```python
from build123d import *

# Parameters (mm, degrees)
SKETCH1_W             = 90
SKETCH1_H             = 90
SKETCH1_R             = 34
BOSS_EXTRUDE1_DEPTH   = 24
SKETCH2_R             = 40.5
CUT_EXTRUDE1_DEPTH    = 16
SKETCH3_R             = 12.7
CUT_EXTRUDE2_DEPTH    = 19
M6X1_0_TAPPED_HOLE1_D = 5
FILLET1_R             = 5
SKETCH7_R             = 30
SKETCH7_R_2           = 20
SKETCH7_R_3           = 12.7
CUT_EXTRUDE3_DEPTH    = 66.620118866
SKETCH8_W             = 13.825432395
SKETCH8_H             = 1
SKETCH8_W_2           = 1
SKETCH8_H_2           = 13.825432395
CUT_EXTRUDE4_DEPTH    = 16


with BuildPart() as part:
    # Sketch1 → Boss-Extrude1 (new body)
    # profile 1 of 2: a face of its own
    with BuildSketch(Plane(origin=(0, 0, 0), x_dir=(1, 0, 0), z_dir=(0, 1, 0))):
        Rectangle(SKETCH1_W, SKETCH1_H)
        Circle(SKETCH1_R, mode=Mode.SUBTRACT)
    # profile 2 of 2: a face of its own
    with BuildSketch(Plane(origin=(0, 0, 0), x_dir=(1, 0, 0), z_dir=(0, 1, 0))):
        Circle(SKETCH1_R)
    extrude(amount=BOSS_EXTRUDE1_DEPTH)

    # Sketch2 → Cut-Extrude1 (cut)
    with BuildSketch(Plane(origin=(0, 24, 0), x_dir=(1, 0, 0), z_dir=(0, 1, 0))):
        with Locations(Location((0, 0, 0), (0, 0, 270))):
            Circle(SKETCH2_R)
    extrude(amount=-CUT_EXTRUDE1_DEPTH, mode=Mode.SUBTRACT)

    # Sketch3 → Cut-Extrude2 (cut)
    with BuildSketch(Plane(origin=(0, 8, 0), x_dir=(1, 0, 0), z_dir=(0, 1, 0))):
        with Locations(Location((0, 0, 0), (0, 0, 270))):
            Circle(SKETCH3_R)
    extrude(amount=-CUT_EXTRUDE2_DEPTH, mode=Mode.SUBTRACT)

    # M6x1.0 Tapped Hole1 (through all)
    with Locations(Plane(origin=(0, 0, 0), x_dir=(-1, 0, 0), z_dir=(0, -1, 0))):
        with Locations((35, 35), (35, -35), (-35, -35), (-35, 35)):
            Hole(M6X1_0_TAPPED_HOLE1_D / 2)

    # Fillet1
    fillet1_edges = [part.edges().sort_by_distance(p)[0] for p in [
        (-45, 12, 45),
        (-45, 12, -45),
        (45, 12, -45),
        (45, 12, 45),
    ]]
    fillet(fillet1_edges, radius=FILLET1_R)

    # Sketch7 → Cut-Extrude3 (cut, through all)
    # profile 1 of 2: a face of its own
    with BuildSketch(Plane(origin=(0, 8, 0), x_dir=(1, 0, 0), z_dir=(0, 1, 0))):
        with Locations(Location((0, 0, 0), (0, 0, 270))):
            Circle(SKETCH7_R)
        Circle(SKETCH7_R_2, mode=Mode.SUBTRACT)
    # profile 2 of 2: a face of its own
    with BuildSketch(Plane(origin=(0, 8, 0), x_dir=(1, 0, 0), z_dir=(0, 1, 0))):
        Circle(SKETCH7_R_2)
        Circle(SKETCH7_R_3, mode=Mode.SUBTRACT)
    extrude(amount=-CUT_EXTRUDE3_DEPTH, mode=Mode.SUBTRACT)

    # Sketch8 → Cut-Extrude4 (cut)
    with BuildSketch(Plane(origin=(0, 24, 0), x_dir=(1, 0, 0), z_dir=(0, 1, 0))):
        with Locations((42.446502967, 0)):
            Rectangle(SKETCH8_W, SKETCH8_H)
        with Locations((0, 42.446502967)):
            Rectangle(SKETCH8_W_2, SKETCH8_H_2)
        with Locations((0, -42.446502967)):
            Rectangle(SKETCH8_W_2, SKETCH8_H_2)
        with Locations((-42.446502967, 0)):
            Rectangle(SKETCH8_W, SKETCH8_H)
    extrude(amount=-CUT_EXTRUDE4_DEPTH, mode=Mode.SUBTRACT)


solid = part.part
```
The listing builds one solid part. Answer for the finished solid, in the listing's coordinates (mm). A direction names the side the tool comes from. Coordinates: 2 decimals unless noted, no trailing zeros. Loops run counter-clockwise (first coordinate to the right, second up) from the corner with the lowest first, then second, coordinate; pieces in that order, holes last. Notation, with made-up numbers: M -14,85.25 L 36,85.25 A26 ccw 36,117.25 Z; hole C 52,48 d2. An arc over 180 degrees is marked long. Answer as a JSON object with one key per item and string values. Group by question number.
Item 1: Each of these flat-tipped pins is pushed along its axis until it touches: P1, Ø1.4, axis at x = 44, y = 16, coming from the -Z side; P2, Ø3.5, axis at y = 13.5, z = -43.5, coming from the -X side; P3, Ø5, axis at x = -43.5, y = 19, coming from the +Z side. Where does it stop, or does it pass through?
Item 2: Section A-A (y = 21.75) is taken. Write down the section's boundary in (x, z).
Item 3: Section B-B (z = 27.5) is taken. Write down the section's boundary in (x, y).
Item 4: Determine the mould class of faces 1 (the face through (1.32, 4.06, -29.97)), 2 (the face through (43, 12, 44)), 3 (the face through (31, 24, -31)) for opening direction Z: +Z half, -Z half, draft (parallel to the pull), parting line (faces both ways), or undercut.
Item 5: Section C-C (x = -35) is taken. Write down the section's boundary in (y, z), and give its area (3 significant figures).
Item 6: Section D-D (x = 16.5) is taken. Write down the section's boundary in (y, z).
Item 7: Consider L1, parallel to Z at x = -35, y = 5; L2, parallel to X at y = 17, z = 35. Determine where each line is inside the solid, lowest interval first.
Item 8: Which of the six approach directions +Z, -Z, +X, -X, +Y, -Y give full straight-line access (tool end or side, diameter ignored) to faces 4 (the face through (-28.946, 16.112, 28.326)), 5 (the face through (-43, 16, -0.5)), 6 (the face through (-0.5, 16, -43))?
Solved:
{
 "1": {"P1": "stops at z = -43.76", "P2": "stops at x = -44.68", "P3": "stops at z = 44.9"},
 "2": {"outline": "M -45,-40 A5 ccw -40,-45 L -0.5,-45 L -0.5,-40.5 A40.5 cw -40.5,-0.5 L -45,-0.5 Z; M -45,0.5 L -40.5,0.5 A40.5 cw -0.5,40.5 L -0.5,45 L -40,45 A5 ccw -45,40 Z; M 0.5,-45 L 40,-45 A5 ccw 45,-40 L 45,-0.5 L 40.5,-0.5 A40.5 cw 0.5,-40.5 Z; M 0.5,40.5 A40.5 cw 40.5,0.5 L 45,0.5 L 45,40 A5 ccw 40,45 L 0.5,45 Z; hole C -35,-35 d5; hole C -35,35 d5; hole C 35,-35 d5; hole C 35,35 d5"},
 "3": {"outline": "M -45,0 L -11.99,0 L -11.99,8 L -29.73,8 L -29.73,24 L -45,24 Z; M 11.99,0 L 45,0 L 45,24 L 29.73,24 L 29.73,8 L 11.99,8 Z"},
 "4": {"face 1": "undercut", "face 2": "+Z half", "face 3": "draft"},
 "5": {"outline": "M 0,-45 L 24,-45 L 24,-37.5 L 0,-37.5 Z; M 0,-32.5 L 24,-32.5 L 24,-20.38 L 8,-20.38 L 8,20.38 L 24,20.38 L 24,32.5 L 0,32.5 Z; M 0,37.5 L 24,37.5 L 24,45 L 0,45 Z", "area": "1,270 mm2"},
 "6": {"outline": "M 0,-45 L 24,-45 L 24,-36.99 L 8,-36.99 L 8,-25.05 L 0,-25.05 Z; M 0,25.05 L 8,25.05 L 8,36.99 L 24,36.99 L 24,45 L 0,45 Z"},
 "7": {"L1": "z = -45 to -37.5, -32.5 to 32.5, 37.5 to 45", "L2": "x = -45 to -37.5, -32.5 to -20.38, 20.38 to 32.5, 37.5 to 45"},
 "8": {"face 4": "+Y", "face 5": "+X, -X, +Y", "face 6": "+Z, -Z, +Y"}
}
